```python
from build123d import *

# Parameters (mm, degrees)
SKETCH1_R                = 19.939
CIRCLE_EXTRUDE_DEPTH     = 6.35
SKETCH3_W                = 6.35
SKETCH3_H                = 39.878
RECTANGLE_EXTRUDE_DEPTH  = 127
SKETCH2_R                = 18.034
CIRCLE_CUT_DEPTH         = 129.712416732
SKETCH6_W                = 125.095
SKETCH6_H                = 36.068
RECTANGLE_CUT_DEPTH      = 129.712416732
SKETCH7_W                = 61.595
SKETCH7_H                = 36.068
END_SHAPE_DEPTH          = 6.35
SKETCH8_R                = 1.905
FOR_SPRING_EXTRUDE_DEPTH = 2.54
MIRRORED_PATTERN_COUNT   = 2
MIRRORED_PATTERN_PITCH   = 254
MIDDLE_CONNECTOR_REACH   = 256.861
SKETCH10_W               = 6.35
SKETCH10_H               = 39.878
SKETCH11_W               = 6.35
SKETCH11_H               = 39.878
END_CUT_DEPTH            = 55.88
SKETCH13_W               = 25.4
SKETCH13_H               = 44.45
BOSS_EXTRUDE1_DEPTH      = 6.35
SKETCH12_W               = 20.066
SKETCH12_H               = 41.148
CUT_EXTRUDE1_DEPTH       = 329.188764629
LPATTERN1_COUNT          = 2
LPATTERN1_PITCH          = 107.188
SKETCH14_R               = 1.55
CUT_EXTRUDE2_DEPTH       = 329.188764629
SKETCH16_W               = 11.43
SKETCH16_H               = 3.302
CUT_EXTRUDE4_DEPTH       = 329.188764629
SKETCH17_W               = 244.663086165
SKETCH17_H               = 85.398325617
SKETCH17_W_2             = 5.588
SKETCH17_H_2             = 39.878
CUT_EXTRUDE5_DEPTH       = 329.188764629


with BuildPart() as part:
    # Sketch1 → circle extrude (new body)
    with BuildSketch(Plane.XY):
        Circle(SKETCH1_R)
    extrude(amount=CIRCLE_EXTRUDE_DEPTH)

    # Sketch3 → rectangle extrude (add)
    with BuildSketch(Plane(origin=(0, 0, 0), x_dir=(0, 0, -1), z_dir=(1, 0, 0))):
        with Locations((-3.175, 0)):
            Rectangle(SKETCH3_W, SKETCH3_H)
    extrude(amount=RECTANGLE_EXTRUDE_DEPTH)

    # Sketch2 → circle cut (cut, through all)
    with BuildSketch(Plane.XY.offset(6.35)):
        Circle(SKETCH2_R)
    extrude(amount=-CIRCLE_CUT_DEPTH, mode=Mode.SUBTRACT)

    # Sketch6 → rectangle cut (cut, through all)
    with BuildSketch(Plane.XY.offset(6.35)):
        with Locations((62.5475, 0)):
            Rectangle(SKETCH6_W, SKETCH6_H)
    extrude(amount=-RECTANGLE_CUT_DEPTH, mode=Mode.SUBTRACT)

    # Sketch7 → end shape (add)
    with BuildSketch(Plane.XY.offset(6.35)):
        with Locations((94.2975, 0)):
            Rectangle(SKETCH7_W, SKETCH7_H)
    extrude(amount=-END_SHAPE_DEPTH)

    # Sketch8 → for spring extrude (add)
    with BuildSketch(Plane.ZY.offset(-63.5)):
        with Locations((3.175, 0)):
            Circle(SKETCH8_R)
    extrude(amount=FOR_SPRING_EXTRUDE_DEPTH)


with BuildPart() as mirrored_pattern_1:
    # mirrored pattern: pattern copy
    add(part.part.moved(Location(Vector(1, 0, 0) * (1 * MIRRORED_PATTERN_PITCH))))

    # Sketch10 → middle connector (add, up to next)
    with BuildSketch(Plane(origin=(127, 0, 0), x_dir=(0, 0, -1), z_dir=(1, 0, 0)), mode=Mode.PRIVATE) as middle_connector_sk1:
        with Locations((-3.175, 0)):
            Rectangle(SKETCH10_W, SKETCH10_H)
    middle_connector_tool1 = extrude(middle_connector_sk1.sketch, amount=MIDDLE_CONNECTOR_REACH, mode=Mode.PRIVATE) - mirrored_pattern_1.part

    add(part.part)  # middle connector merges part
    add(middle_connector_tool1.solids().sort_by_distance((127, 0, 3.175))[0])

    # Sketch11 → end cut (cut)
    with BuildSketch(Plane(origin=(381, 0, 0), x_dir=(0, 0, -1), z_dir=(1, 0, 0))):
        with Locations((-3.175, 0)):
            Rectangle(SKETCH11_W, SKETCH11_H)
    extrude(amount=-END_CUT_DEPTH, mode=Mode.SUBTRACT)

    # Sketch13 → Boss-Extrude1 (add)
    with BuildSketch(Plane.XY.offset(6.35)):
        with Locations((215.9, -22.098)):
            Rectangle(SKETCH13_W, SKETCH13_H)
    boss_extrude1 = extrude(amount=-BOSS_EXTRUDE1_DEPTH)

    # Sketch12 → Cut-Extrude1 (cut, through all)
    with BuildSketch(Plane.XY.offset(6.35)):
        with Locations((216.027, -20.447)):
            Rectangle(SKETCH12_W, SKETCH12_H)
    cut_extrude1 = extrude(amount=-CUT_EXTRUDE1_DEPTH, mode=Mode.SUBTRACT)

    # LPattern1: Boss-Extrude1, Cut-Extrude1 ×2
    with Locations(*[(-i * LPATTERN1_PITCH, 0, 0) for i in range(1, LPATTERN1_COUNT)]):
        add(boss_extrude1)
        add(cut_extrude1, mode=Mode.SUBTRACT)

    # Sketch14 → Cut-Extrude2 (cut, through all)
    with BuildSketch(Plane(origin=(0, 0, 0), x_dir=(-1, 0, 0), z_dir=(0, 0, -1))):
        with Locations((-103.96, 3.88)):
            Circle(SKETCH14_R)
        with Locations((-113.96, 3.88)):
            Circle(SKETCH14_R)
        with Locations((-211.021, 3.88)):
            Circle(SKETCH14_R)
        with Locations((-221.021, 3.88)):
            Circle(SKETCH14_R)
    extrude(amount=-CUT_EXTRUDE2_DEPTH, mode=Mode.SUBTRACT)

    # Sketch16 → Cut-Extrude4 (cut, through all)
    with BuildSketch(Plane.XY.offset(6.35)):
        with Locations((216.027, -42.672)):
            Rectangle(SKETCH16_W, SKETCH16_H)
    extrude(amount=-CUT_EXTRUDE4_DEPTH, mode=Mode.SUBTRACT)

    # Sketch17 → Cut-Extrude5 (cut, through all)
    with BuildSketch(Plane.XY.offset(6.35)):
        with Locations((75.534456918, -9.69861823)):
            Rectangle(SKETCH17_W, SKETCH17_H)
        with Locations((322.326, 0)):
            Rectangle(SKETCH17_W_2, SKETCH17_H_2)
    extrude(amount=-CUT_EXTRUDE5_DEPTH, mode=Mode.SUBTRACT)


solid = mirrored_pattern_1.part
```
Input: part model. Units: mm. Frame: model coordinates. A direction names the side the tool comes from. Give positions to 0.01 mm unless a question says otherwise; leave off trailing zeros. Loops run counter-clockwise (first coordinate to the right, second up) from the corner with the lowest first, then second, coordinate; pieces in that order, holes last. Notation, with made-up numbers: M -25,58.5 L -12,58.5 A23 cw -12,89.5 Z; hole C -3,-39 d4. An arc over 180 degrees is marked long. Answer as CSV lines item,"result". Start each with the question number.
1. Section C-C on z = 3. Return loops of the section in (x, y).
2. Reachability of faces 1 (the face through (210.312, -43, 3)), 2 (the face through (235.97, 0.4, 3.22)), 3 (the face through (203.2, -32, 3)), 4 (the face through (228.6, -32, 3)) from +Z, -Z, +X, -X, +Y, -Y: full face, straight path, thin tool, end or side. Return the list, or none.
3. Pull-direction query (X, two-part tool) for faces 5 (the face through (208, -41.021, 3)), 6 (the face through (231, -3, 0)), 7 (the face through (319.532, 0, 3)); classes: released by +X, released by -X, zero draft, split by the parting line, or undercut.
4. Section D-D on y = 3.88. Return loops of the section in (x, z).
5. Pin query (flat end, axial travel): P1, Ø3.5, axis at y = -42, z = 4, coming from the -X side; P2, Ø1.9, axis at x = 279, z = 4.5, coming from the -Y side; P3, Ø1.7, axis at y = -42.5, z = 2, coming from the +X side. Return the tip coordinate at first contact, or that it passes through.
6. Section B-B on y = -36. Return loops of the section in (x, z), plus the area to 3 significant figures.
7. Section A-A on x = 280. Return loops of the section in (y, z), plus the area to 3 significant figures.
8. Line query: L1, parallel to X at y = -31, z = 1; L2, parallel to Y at x = 283, z = 0.5; L3, parallel to X at y = -16.5, z = 5.75. Output: solid intervals per line, ascending.
Computed values:
1,outline,"M 197.87,-19.94 L 203.2,-19.94 L 203.2,-44.32 L 210.31,-44.32 L 210.31,-41.02 L 205.99,-41.02 L 205.99,0.13 L 226.06,0.13 L 226.06,-41.02 L 221.74,-41.02 L 221.74,-44.32 L 228.6,-44.32 L 228.6,-19.94 L 319.53,-19.94 L 319.53,19.94 L 197.87,19.94 Z; hole C 211.02,3.88 d3.1; hole C 221.02,3.88 d3.1; hole M 254,-18.03 L 317.5,-18.03 L 317.5,-1.9 L 314.96,-1.9 L 314.96,1.9 L 317.5,1.9 L 317.5,18.03 L 254,18.03 A18.03 ccw Z"
2,face 1,"+Z, -Z, -Y"
2,face 2,"+Z, -Z"
2,face 3,"+Z, -Z, -X, -Y"
2,face 4,"+Z, -Z, +X, -Y"
3,face 5,"undercut"
3,face 6,"zero draft"
3,face 7,"released by +X"
4,outline,"M 197.87,0 L 209.47,0 L 209.47,6.35 L 197.87,6.35 Z; M 212.57,0 L 219.47,0 L 219.47,6.35 L 212.57,6.35 Z; M 222.57,0 L 236.39,0 L 236.39,6.35 L 222.57,6.35 Z; M 317.5,0 L 319.53,0 L 319.53,6.35 L 317.5,6.35 Z"
5,P1,"stops at x = 203.2"
5,P2,"stops at y = -19.94"
5,P3,"stops at x = 228.6"
6,outline,"M 203.2,0 L 205.99,0 L 205.99,6.35 L 203.2,6.35 Z; M 226.06,0 L 228.6,0 L 228.6,6.35 L 226.06,6.35 Z"
6,area,"33.9 mm²"
7,outline,"M -19.94,0 L -18.03,0 L -18.03,6.35 L -19.94,6.35 Z; M 18.03,0 L 19.94,0 L 19.94,6.35 L 18.03,6.35 Z"
7,area,"24.2 mm²"
8,L1,"x = 203.2 to 205.99, 226.06 to 228.6"
8,L2,"y = -19.94 to -18.03, 18.03 to 19.94"
8,L3,"x = 197.87 to 205.99, 226.06 to 246.72, 317.5 to 319.53"
